Input: dimensioned drawing with shaded views. Units: mm. Origin: part minimum x, y, z. A direction names the side the tool comes from. Round coordinates to 2 decimals unless told otherwise and drop trailing zeros. Order: outer loops, then holes, each group sorted by start corner. A loop starts at its lowest first (then second) coordinate and runs counter-clockwise, first axis right, second up. Notation, with made-up numbers: (-28.75, -18.75) -> (15.25, -18.75) arc R11 ccw to (15.25, -12.75) -> close; hole circle Ø10 at (67, 19.5). An arc over 180 degrees is marked (long way). Use a Markdown table: item, result. Add a question column.
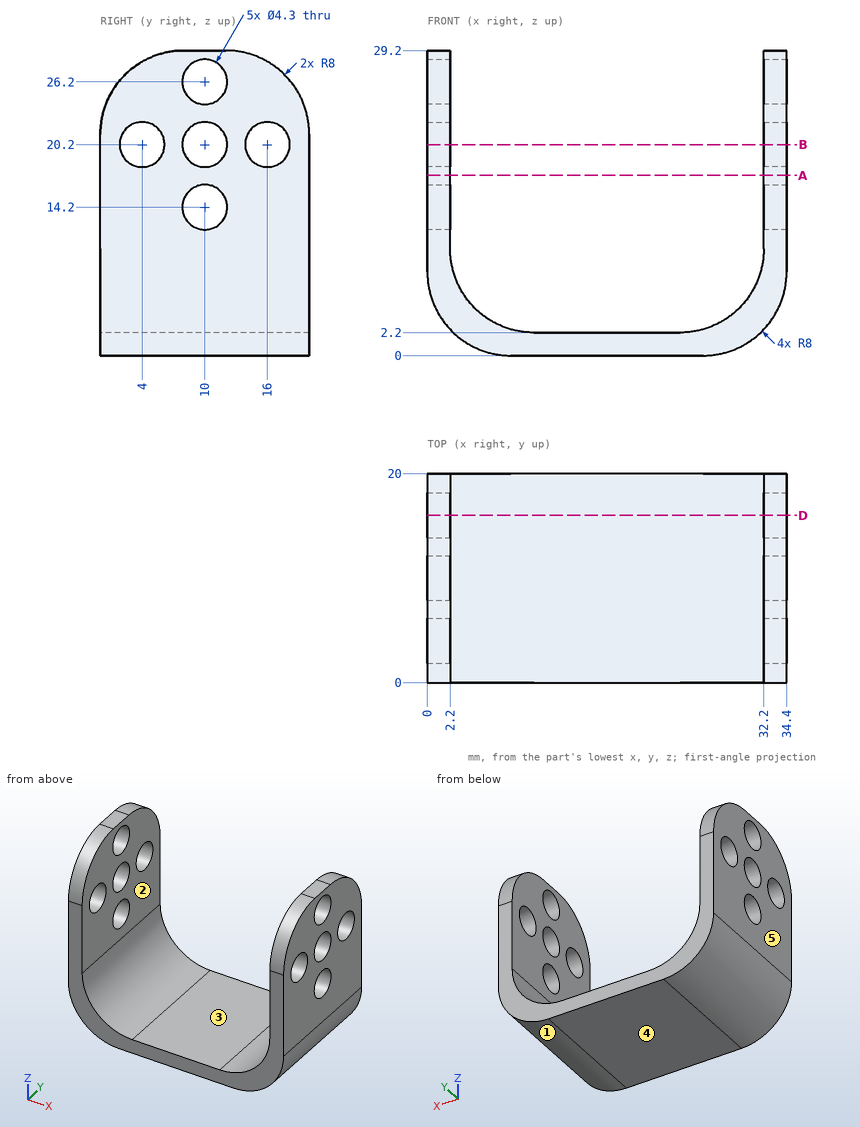
1) Draft query along X for the marked faces 3, 4 and 5. Return one class per face: pulls with the +X half, pulls with the -X half, needs draft (parallel to the pull), parting line crosses it, or undercut.
2) Section B-B on z = 20.2. Count the separate pieces of the cut face and the enclosed holes in it, then the cut area to 3 significant figures.
3) Reachability of the marked faces 1 and 2 from +Z, -Z, +X, -X, +Y, -Y: full face, straight path, thin tool, end or side. Return the list, or none.
4) Line query: probe 1 along Y at (x, z) = (0.8, 20.2); probe 2 along X at (y, z) = (3, 25.75); probe 3 along Z at (x, y) = (1.5, 11.25). Output: solid intervals per line, ascending. Write a range as from..to.
5) Section A-A on z = 17.25. Output: boundary loops of the cut face in (x, y), then the cut area to 3 significant figures.
6) First-contact query: pin 1 Ø8 at (x, z) = (8, 4.5) entering from +Y; pin 2 Ø7 at (x, y) = (20.5, 10) entering from +Z; pin 3 Ø1.5 at (y, z) = (5.5, 7) entering from +X. Flat tips, straight axial feed; report the tip coordinate or a pass-through.
7) Section D-D on y = 16. Output: boundary loops of the cut face in (x, z), then the cut area to 3 significant figures.
Conclusion:
| question | item | result |
|---|---|---|
| 1 | face 3 | undercut |
| 1 | face 4 | needs draft |
| 1 | face 5 | pulls with the -X half |
| 2 | separate pieces | 8 |
| 2 | enclosed holes | 0 |
| 2 | area | 31.2 mm^2 |
| 3 | face 1 | -Z, +X, +Y, -Y |
| 3 | face 2 | +Z, +Y, -Y |
| 4 | probe 1 | y = 0..1.85, 6.15..7.85, 12.15..13.85, 18.15..20 |
| 4 | probe 2 | x = 0..2.2, 32.2..34.4 |
| 4 | probe 3 | z = 3.34..12.45, 15.95..18.45, 21.95..24.45, 27.95..29.2 |
| 5 | outline | (0, 0) -> (2.2, 0) -> (2.2, 20) -> (0, 20) -> close; (32.2, 0) -> (34.4, 0) -> (34.4, 20) -> (32.2, 20) -> close |
| 5 | area | 88.0 mm^2 |
| 6 | pin 1 | stops at y = 20 |
| 6 | pin 2 | stops at z = 2.2 |
| 6 | pin 3 | stops at x = 34.4 |
| 7 | outline | (0, 8) arc R8 ccw to (8, 0) -> (26.4, 0) arc R8 ccw to (34.4, 8) -> (34.4, 18.05) -> (32.2, 18.05) -> (32.2, 10.2) arc R8 cw to (24.2, 2.2) -> (10.2, 2.2) arc R8 cw to (2.2, 10.2) -> (2.2, 18.05) -> (0, 18.05) -> close; (0, 22.35) -> (2.2, 22.35) -> (2.2, 28.13) -> (0, 28.13) -> close; (32.2, 22.35) -> (34.4, 22.35) -> (34.4, 28.13) -> (32.2, 28.13) -> close |
| 7 | area | 171 mm^2 |
